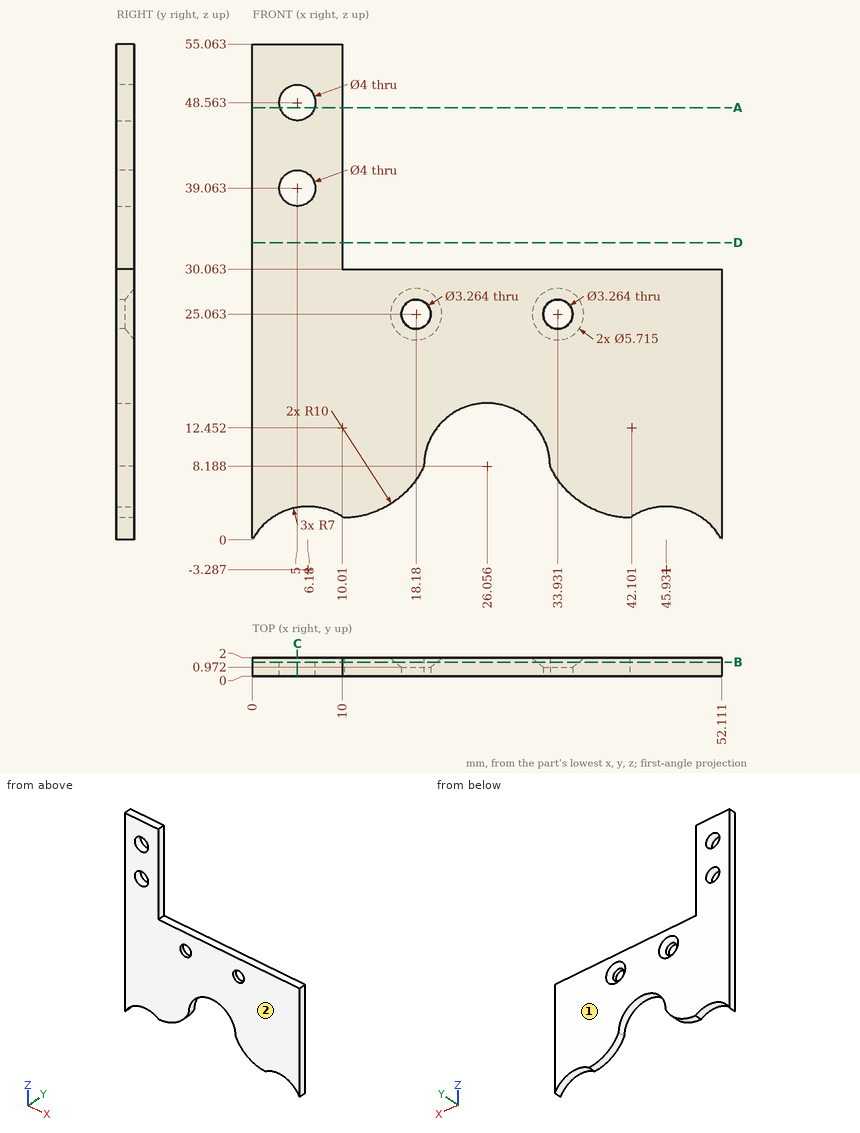
Geometry check sheet. Reference: drawing and pictorial views, mm from the part's lowest x, y, z. Give positions to 0.01 mm unless a question says otherwise; leave off trailing zeros. Order: outer loops, then holes, each group sorted by start corner. A loop starts at its lowest first (then second) coordinate and runs counter-clockwise, first axis right, second up. Notation, with made-up numbers: (-15, -32) - (41, -32) arc R13 cw to (41, -18) - close; hole circle Ø11 at (8, -3). An arc over 180 degrees is marked (long way). Answer as CSV lines item,"result". Start each with the question number.
Item 1: Mould release check, pull along Y, two halves, no side actions. Record for the marked faces 1 and 2: released by +Y, released by -Y, zero draft, split by the parting line, or undercut.
Item 2: Material ranges on L1, parallel to X at y = 1, z = 2 (1 decimal); L2, parallel to X at y = 0.5, z = 51.5; L3, parallel to X at y = 1.8, z = 12 (1 decimal), recorded low to high.
Item 3: Section check A-A, the plane z = 48. Record the boundary of the cut face in (x, y), plus the area to 3 significant figures.
Item 4: Section check D-D, the plane z = 33. Record the boundary of the cut face in (x, y), plus the area to 3 significant figures.
Item 5: Section check B-B, the plane y = 1.55. Record the boundary of the cut face in (x, z) (1 decimal).
Item 6: Gauge pin test, flat ends, axial feed: pin 1 (5 mm diameter, centred on x = 15.5, z = 33, fed in from -Y); pin 2 (1 mm diameter, centred on y = 1, z = 49, fed in from +X); pin 3 (0.6 mm diameter, centred on x = 37.5, y = 1.5, fed in from +Z). Record the tip position at first contact, or that the pin passes through.
Item 7: Section check C-C, the plane x = 5. Record the boundary of the cut face in (y, z).
Filled in:
1,face 1,"released by +Y"
1,face 2,"released by -Y"
2,L1,"0 to 1.6, 50.5 to 52.1"
2,L2,"0 to 10"
2,L3,"0 to 20.2, 31.9 to 52.1"
3,outline,"(0, 0) - (3.08, 0) - (3.08, 2) - (0, 2) - close; (6.92, 0) - (10, 0) - (10, 2) - (6.92, 2) - close"
3,area,"12.3 mm^2"
4,outline,"(0, 0) - (10, 0) - (10, 2) - (0, 2) - close"
4,area,"20.0 mm^2"
5,outline,"(0, 0) arc R7 cw to (10.2, 2.5) arc R10 ccw to (19.1, 8.2) arc R7 cw to (33.1, 8.2) arc R10 ccw to (41.9, 2.5) arc R7 cw to (52.1, 0) - (52.1, 30.1) - (10, 30.1) - (10, 55.1) - (0, 55.1) - close; hole circle Ø4 at (5, 39.1); hole circle Ø4 at (5, 48.6); hole circle Ø4.6 at (18.2, 25.1); hole circle Ø4.6 at (33.9, 25.1)"
6,pin 1,"through"
6,pin 2,"x = 10"
6,pin 3,"z = 30.06"
7,outline,"(0, 3.61) - (2, 3.61) - (2, 37.06) - (0, 37.06) - close; (0, 41.06) - (2, 41.06) - (2, 46.56) - (0, 46.56) - close; (0, 50.56) - (2, 50.56) - (2, 55.06) - (0, 55.06) - close"
